Source: CAD feature listing. Evaluate the final solid. Frame: model axes, mm. A direction names the side the tool comes from. Coordinates: 2 decimals unless noted, no trailing zeros. Order: outer loops, then holes, each group sorted by start corner. A loop starts at its lowest first (then second) coordinate and runs counter-clockwise, first axis right, second up.
Item 1: Section D-D on x = 30. Return the cut outline in (y, z).
Item 2: Reachability of faces 4 (the flat face through (111, 1, 85)), 5 (the flat face through (116, -85, 42)), 6 (the cylindrical face through (-117, 15, 20)) from +Z, -Z, +X, -X, +Y, -Y: full face, straight path, thin tool, end or side. Return the list, or none.
Item 3: Section B-B on z = 65. Return the cut outline in (x, y).
Item 4: Mould query, pull axis Y, two halves, no side actions, for faces 1 (the flat face through (-117.5, -1, 43)), 2 (the flat face through (2, 85, 6)), 3 (the cylindrical face through (-117, -15, 20)). Classes: released by +Y, released by -Y, zero draft, split by the parting line, or undercut.
Item 5: Section C-C on y = -60. Return the cut outline in (x, z), then the cut area to 3 significant figures.
Item 6: Section A-A on z = 42. Return the cut outline in (x, y), then the cut area to 3 significant figures.
Item 7: Ray query, line 1 (Z direction, x = 104, y = 83.95); line 2 (X direction, y = -55, z = 32.5); line 3 (Z direction, x = -1.5, y = 41.5). Return the intervals inside material, ascending.
Item 8: Contact query for flat-ended pins moving along their axis: P1, Ø0.6, axis at x = -117, y = 6.5, coming from the -Z side; P2, Ø0.6, axis at x = 46, y = 84, coming from the +Z side; P3, Ø5, axis at x = -77.5, y = -55.5, coming from the +Z side. Output: stop coordinate, or through.
from build123d import *

# Parameters (mm, degrees)
F1_DEPTH  = 2
F2_W      = 2
F2_H      = 170
F3_DEPTH  = 83
F4_R      = 1
F5_W      = 10
F5_H      = 166
F6_DEPTH  = 2
F7_R      = 1
F8_W      = 224
F8_H      = 2
F9_DEPTH  = 9
F10_R     = 1
F11_W     = 0.5
F11_H     = 1
F12_DEPTH = 235.001
F14_DEPTH = 3
F15_R     = 1.2
F16_DEPTH = 170.001


with BuildPart() as f1:
    # F0 (on Top) → F1 (new body)
    with BuildSketch(Plane.XY):
        Polygon((112.5, -85), (117.5, -85), (117.5, 85), (112.5, 85), (112.5, 82), (112, 82), (112, 85), (-112, 85), (-112, 82), (-112.5, 82), (-112.5, 85), (-117.5, 85), (-117.5, -85), (-112.5, -85), (-112.5, -82), (-112, -82), (-112, -85), (112, -85), (112, -82), (112.5, -82), align=None)
    extrude(amount=F1_DEPTH)

    # F2 (on face) → F3 (join)
    with BuildSketch(Plane.XY.offset(2)):
        with Locations((116.5, 0)):
            Rectangle(F2_W, F2_H)
        with Locations((-116.5, 0)):
            Rectangle(F2_W, F2_H)
    extrude(amount=F3_DEPTH)

    # F4
    f4_edges = [f1.edges().sort_by_distance(p)[0] for p in [
        (-117.5, 0, 0),
        (117.5, 0, 0),
        (-115.5, 0, 2),
        (115.5, 0, 2),
    ]]
    fillet(f4_edges, radius=F4_R)

    # F5 (on face) → F6 (join)
    with BuildSketch(Plane.XY.offset(85)):
        with Locations((-112.5, 0)):
            Rectangle(F5_W, F5_H)
        with Locations((112.5, 0)):
            Rectangle(F5_W, F5_H)
    extrude(amount=F6_DEPTH)

    # F7
    f7_edges = [f1.edges().sort_by_distance(p)[0] for p in [
        (-117.5, 0, 87),
        (117.5, 0, 87),
        (-115.5, 0, 85),
        (115.5, 0, 85),
    ]]
    fillet(f7_edges, radius=F7_R)

    # F8 (on face) → F9 (join)
    with BuildSketch(Plane.XY.offset(2)):
        with Locations((0, -84)):
            Rectangle(F8_W, F8_H)
        with Locations((0, 84)):
            Rectangle(F8_W, F8_H)
    extrude(amount=F9_DEPTH)

    # F10
    f10_edges = [f1.edges().sort_by_distance(p)[0] for p in [
        (0, -85, 0),
        (0, -83, 2),
        (0, 83, 2),
        (0, 85, 0),
    ]]
    fillet(f10_edges, radius=F10_R)

    # F11 (on face) → F12 (cut, through all)
    with BuildSketch(Plane(origin=(-117.5, 0, 0), x_dir=(0, -1, 0), z_dir=(-1, 0, 0))):
        with Locations((83.25, 84.5)):
            Rectangle(F11_W, F11_H)
        with Locations((-83.25, 84.5)):
            Rectangle(F11_W, F11_H)
    extrude(amount=-F12_DEPTH, mode=Mode.SUBTRACT)

    # F13 (on face) → F14 (cut)
    with BuildSketch(Plane(origin=(-117.5, 0, 0), x_dir=(0, -1, 0), z_dir=(-1, 0, 0))):
        with BuildLine():
            Line((-7.5, 12.5), (7.5, 12.5))
            ThreePointArc((7.5, 12.5), (15, 20), (7.5, 27.5))
            Line((7.5, 27.5), (-7.5, 27.5))
            ThreePointArc((-7.5, 27.5), (-15, 20), (-7.5, 12.5))
        make_face()
        with BuildLine():
            Line((-15, 55), (15, 55))
            ThreePointArc((15, 55), (25, 65), (15, 75))
            Line((15, 75), (-15, 75))
            ThreePointArc((-15, 75), (-25, 65), (-15, 55))
        make_face()
    extrude(amount=-F14_DEPTH, mode=Mode.SUBTRACT)

    # F15 (on face) → F16 (cut, through all)
    with BuildSketch(Plane.XZ.offset(85)):
        with Locations((104, 7)):
            Circle(F15_R)
        with Locations((-104, 7)):
            Circle(F15_R)
    extrude(amount=-F16_DEPTH, mode=Mode.SUBTRACT)


solid = f1.part
Answer list:
1. outline: (-85, 1) arc R1 ccw to (-84, 0) - (84, 0) arc R1 ccw to (85, 1) - (85, 11) - (83, 11) - (83, 3) arc R1 cw to (82, 2) - (-82, 2) arc R1 cw to (-83, 3) - (-83, 11) - (-85, 11) - close
2. face 4: +Y, -Y
2. face 5: +Z, -Z, +X, -X, -Y
2. face 6: -X
3. outline: (-117.5, -85) - (-115.5, -85) - (-115.5, -25) - (-117.5, -25) - close; (-117.5, 25) - (-115.5, 25) - (-115.5, 85) - (-117.5, 85) - close; (115.5, -85) - (117.5, -85) - (117.5, 85) - (115.5, 85) - close
4. face 1: zero draft
4. face 2: released by +Y
4. face 3: undercut
5. outline: (-117.5, 1) arc R1 ccw to (-116.5, 0) - (116.5, 0) arc R1 ccw to (117.5, 1) - (117.5, 86) arc R1 ccw to (116.5, 87) - (107.5, 87) - (107.5, 85) - (114.5, 85) arc R1 cw to (115.5, 84) - (115.5, 3) arc R1 cw to (114.5, 2) - (-114.5, 2) arc R1 cw to (-115.5, 3) - (-115.5, 84) arc R1 cw to (-114.5, 85) - (-107.5, 85) - (-107.5, 87) - (-116.5, 87) arc R1 ccw to (-117.5, 86) - close
5. area: 842 mm2
6. outline: (-117.5, -85) - (-115.5, -85) - (-115.5, 85) - (-117.5, 85) - close; (115.5, -85) - (117.5, -85) - (117.5, 85) - (115.5, 85) - close
6. area: 680 mm2
7. line 1: z = 0 to 5.8, 8.2 to 11
7. line 2: x = -117.5 to -115.5, 115.5 to 117.5
7. line 3: z = 0 to 2
8. P1: stops at z = 0.02
8. P2: stops at z = 11
8. P3: stops at z = 2
